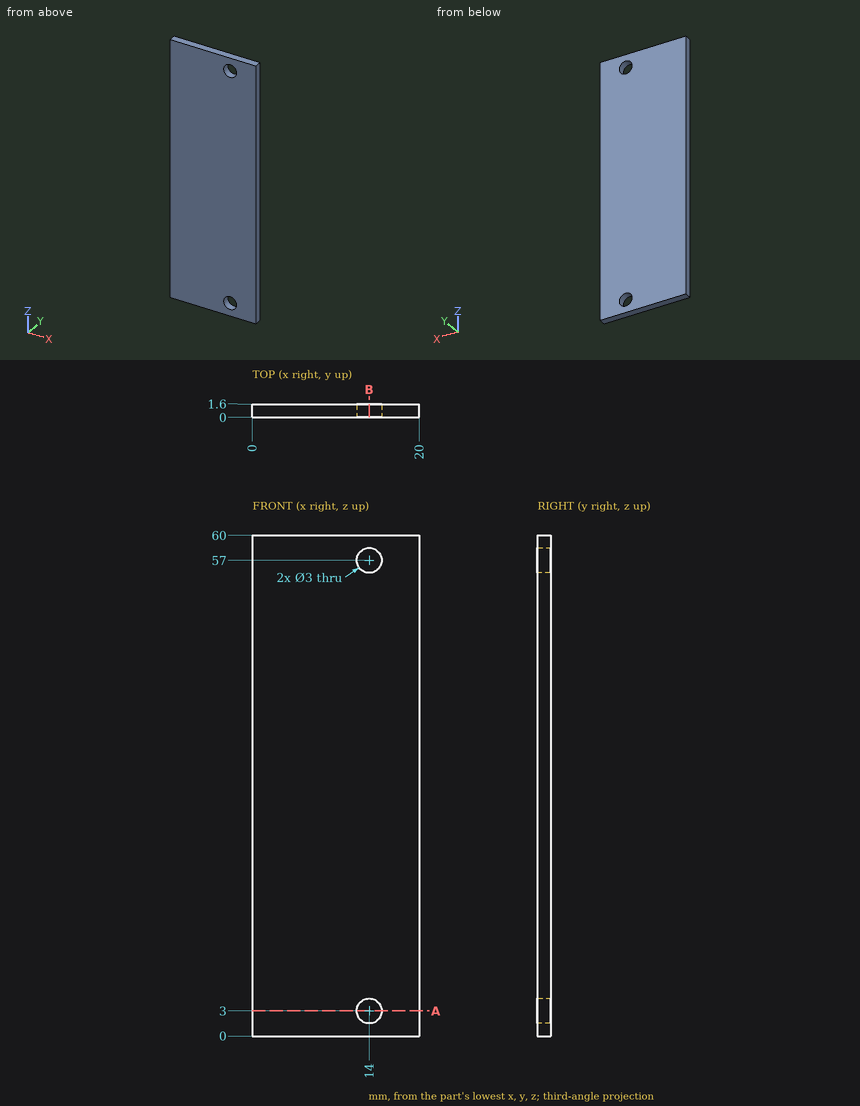
Source: three-view drawing plus pictorial views. Frame: mm from the lowest corner of the part. Give positions to 0.01 mm unless a question says otherwise; leave off trailing zeros. Order: outer loops, then holes, each group sorted by start corner. A loop starts at its lowest first (then second) coordinate and runs counter-clockwise, first axis right, second up. Notation, with made-up numbers: M 31.5,-35.5 L 70.5,-35.5 A14 cw 70.5,-22.5 Z; hole C -11,-7 d3. An arc over 180 degrees is marked long. One line per question, with ' | ' between items.
1) Section B-B on x = 14. Output: boundary loops of the cut face in (y, z), and give its area (3 significant figures).
Filled in:
outline: M 0,0 L 1.6,0 L 1.6,1.5 L 0,1.5 Z; M 0,4.5 L 1.6,4.5 L 1.6,55.5 L 0,55.5 Z; M 0,58.5 L 1.6,58.5 L 1.6,60 L 0,60 Z | area: 86.4 mm2
2) Section A-A on z = 3. Output: boundary loops of the cut face in (x, y).
Filled in:
outline: M 0,0 L 12.5,0 L 12.5,1.6 L 0,1.6 Z; M 15.5,0 L 20,0 L 20,1.6 L 15.5,1.6 Z
3) Ray query, L1, parallel to Z at x = 13.25, y = 0.9; L2, parallel to X at y = 1.2, z = 3; L3, parallel to Z at x = 14.25, y = 0.15. Return the intervals inside material, ascending.
Filled in:
L1: z = 0 to 1.7, 4.3 to 55.7, 58.3 to 60 | L2: x = 0 to 12.5, 15.5 to 20 | L3: z = 0 to 1.52, 4.48 to 55.52, 58.48 to 60
